Autodesk Inventor part; units mm, degrees
ref_plane "YZ Plane" through (0, 0, 0) normal (1, 0, 0) x (0, 1, 0)
ref_plane "XZ Plane" through (0, 0, 0) normal (0, 1, 0) x (-1, 0, 0)
ref_plane "XY Plane" through (0, 0, 0) normal (0, 0, 1) x (1, 0, 0)
sketch "Skizze1" plane through (0, 0, 0) normal (0, 1, 0) x (-1, 0, 0)
  line L0 (20.5, -10.1) -> (-20.5, -10.1)
  line L1 (-20.5, -10.1) -> (-20.5, 10.1)
  line L2 (-20.5, 10.1) -> (20.5, 10.1)
  line L3 (20.5, 10.1) -> (20.5, -10.1)
  line L4 (0, -23.94) -> (0, 23.94)
  line L5 (-40.6, 0) -> (40.6, 0)
  line L6 (29, -17.1) -> (-29, -17.1)
  line L7 (-29, -17.1) -> (-29, 17.1)
  line L8 (-29, 17.1) -> (29, 17.1)
  line L9 (29, 17.1) -> (29, -17.1)
  point P0 (0, 0)
  dimension "d0" = 41
  dimension "d3" = 20.2
  dimension "d7" = 58
  dimension "d8" = 7
extrude "Extrusion2" add sketch "Skizze1" along normal mid plane 4 contours L3 L5 L9 L6 L4 L0 | L4 L6 L7 L5 L1 L0 | L3 L2 L4 L8 L9 L5 | L5 L7 L8 L4 L2 L1
sketch "Skizze2" plane through (0, 2, 0) normal (0, 1, 0) x (1, 0, 0)
  circle A0 centre (-24, 5) radius 1.6
  circle A1 centre (-24, -5) radius 1.6
  line L0 (-29, 17.1) -> (-29, -17.1)
  line L1 (40.6, 0) -> (-40.6, 0)
  line L2 (0, 23.94) -> (0, -23.94)
  circle A2 centre (24, 5) radius 1.6
  circle A3 centre (24, -5) radius 1.6
  line L3 (-20.5, -10.1) -> (-20.5, 10.1)
  point P0 (0, 0)
  dimension "d11" = 3.2
  dimension "d12" = 3.2
  dimension "d15" = 10
  dimension "d16" = 5
  dimension "d58" = 3.5
  dimension "d59" = 3.5
extrude "Extrusion3" cut sketch "Skizze2" against normal up to surface (4 mm away)
sketch "Skizze3" plane through (0, 2, 0) normal (0, 1, 0) x (1, 0, 0)
  line L0 (-20.5, -10.1) -> (-20.5, 10.1)
  line L1 (-20.5, -0.75) -> (-27.5, -0.75)
  line L2 (-27.5, -0.75) -> (-27.5, 0.75)
  line L3 (-27.5, 0.75) -> (-20.5, 0.75)
  line L4 (-20.5, 0.75) -> (-20.5, -0.75)
  line L5 (40.6, 0) -> (-40.6, 0)
  line L6 (0, 23.94) -> (0, -23.94)
  line L7 (20.5, 10.1) -> (20.5, -10.1)
  line L8 (20.5, 0.75) -> (27.5, 0.75)
  line L9 (27.5, 0.75) -> (27.5, -0.75)
  line L10 (27.5, -0.75) -> (20.5, -0.75)
  line L11 (20.5, -0.75) -> (20.5, 0.75)
  point P0 (0, 0)
  dimension "d19" = 7
  dimension "d20" = 1.5
  dimension "d23" = 7
extrude "Extrusion4" cut sketch "Skizze3" against normal blind 2 contours L1 L2 L5 L0 | L5 L2 L3 L0
extrude "Extrusion5" cut sketch "Skizze3" against normal blind 2 contours L9 L10 L7 L5 | L5 L7 L8 L9
sketch "Skizze4" plane through (0, 0, 0) normal (0, 0, 1) x (1, 0, 0)
  line L0 (0, 34.5995) -> (0, -8.0999)
  line L1 (-12.8217, 0) -> (76.93, 0)
  line L2 (29, 2) -> (29, -2)
  line L3 (29, -2) -> (32, -2)
  line L4 (32, -2) -> (32, 19.216)
  line L5 (32, 19.216) -> (29, 19.216)
  line L6 (29, 19.216) -> (29, -2)
  line L7 (32, -2) -> (50.7939, 4.8404)
  line L8 (50.7939, 4.8404) -> (50.7939, 26.0564)
  line L9 (50.7939, 26.0564) -> (32, 19.216)
  line L10 (32, 15.858) -> (48.1939, 21.7521)
  line L11 (48.0492, 7.1994) -> (32, 1.358)
  line L12 (48.1939, 21.7521) -> (65.1083, 27.9084)
  line L13 (65.1083, 27.9084) -> (65.1083, 13.4084)
  line L14 (65.1083, 13.4084) -> (48.0492, 7.1994)
  line L15 (50.7939, 15.4484) -> (37.5768, 10.6378)
  line L16 (50.7939, 15.4484) -> (64.8591, 15.4484) construction
  point P0 (0, 0)
  point P1 (50.7939, 22.6984)
  point P2 (50.7939, 8.1984)
  dimension "d26" = 3
  dimension "d27" = 21.216
  dimension "d28" = 20
  dimension "d29" = 21.216
  dimension "d30" = 20
  dimension "d38" = 110
  dimension "d42" = 18
  dimension "d44" = 110
  dimension "d48" = 14.3145
  dimension "d66" = 14.5
  dimension "d67" = 160
extrude "Extrusion6" add sketch "Skizze4" along normal mid plane 34.2 contours L2 L6 L5 L4 L1 | L1 L4 L3 L2
sketch "Skizze6" plane through (0, 0, 0) normal (0, 0, 1) x (1, 0, 0)
  point P0 (0, 0)
extrude "Extrusion7" add sketch "Skizze4" along normal mid plane 20 contours L4 L11 L14 L8 L7 L1 | L1 L7 L4 | L4 L10 L12 L8 L14 L11 | L4 L9 L8 L12 L10
extrude "Extrusion9" add sketch "Skizze4" along normal mid plane 13.5 contours L8 L12 L13 L14
shell "Wandung2" thickness 2 removed faces 1 at (65.1083, 18.2418, -2.25)
fillet "Rundung1" radius 4 4 edges at (41.3969, 22.6362, 10) (41.3969, 22.6362, -10) (41.3969, 1.4202, -10) (41.3969, 1.4202, 10)
sketch "Skizze7" plane through (-29, -2, 17.1) normal (0, 0, 1) x (1, 0, 0)
  line L0 (-12.2, 2) -> (73.2, 2)
  line L1 (29, 25.4592) -> (29, -4.2432)
  line L2 (58, 4) -> (58, 21.216)
  line L3 (58, 21.216) -> (29, 4)
  line L4 (8.5, 4) -> (49.5, 4)
  line L5 (58, 4) -> (0, 4)
  line L6 (58, 4) -> (58, 21.216)
  point P0 (29, 2)
extrude "Extrusion10" add sketch "Skizze7" against normal blind 2
sketch "Skizze8" plane through (-29, -2, -17.1) normal (0, 0, -1) x (-1, 0, 0)
  line L0 (-29, -4.2432) -> (-29, 25.4592)
  line L1 (-73.2, 2) -> (12.2, 2)
  line L2 (-58, 4) -> (-58, 21.216)
  line L3 (-58, 21.216) -> (-29, 4)
  line L4 (-8.5, 4) -> (-49.5, 4)
  line L5 (-58, 4) -> (0, 4)
  line L6 (-58, 21.216) -> (-61, 21.216)
  line L7 (-58, 4) -> (-58, 21.216)
  point P0 (-29, 2)
extrude "Extrusion11" add sketch "Skizze8" against normal blind 2
sketch "Skizze9" plane through (0, 0, 6.75) normal (0, 0, 1) x (1, 0, 0)
  circle A0 centre (58.7939, 18.3602) radius 1.6
  line L0 (65.1083, 13.4084) -> (65.1083, 27.9084)
  line L1 (65.1083, 15.5368) -> (65.1083, 25.7801)
  line L2 (65.1083, 20.6584) -> (53.7155, 16.5118)
  line L3 (65.1083, 20.6584) -> (77.2323, 20.6584) construction
  line L4 (50.7939, 8.1984) -> (50.7939, 22.6984)
  point P0 (0, 0)
  dimension "d60" = 3.2
  dimension "d62" = 160
  dimension "d63" = 8
extrude "Extrusion12" cut sketch "Skizze9" against normal up to surface (13.5 mm away)
sketch "Skizze10" plane through (0, 0, 0) normal (0, 0, 1) x (1, 0, 0)
  line L0 (-46.9108, 47.129) -> (37.4559, 47.129)
  line L1 (37.4559, 47.129) -> (37.4559, -27.201)
  line L2 (37.4559, -27.201) -> (-46.9108, -27.201)
  line L3 (-46.9108, -27.201) -> (-46.9108, 47.129)
  point P0 (0, 0)
extrude "Extrusion13" cut sketch "Skizze10" along normal mid plane 50
properties part number "_3D-Druck"
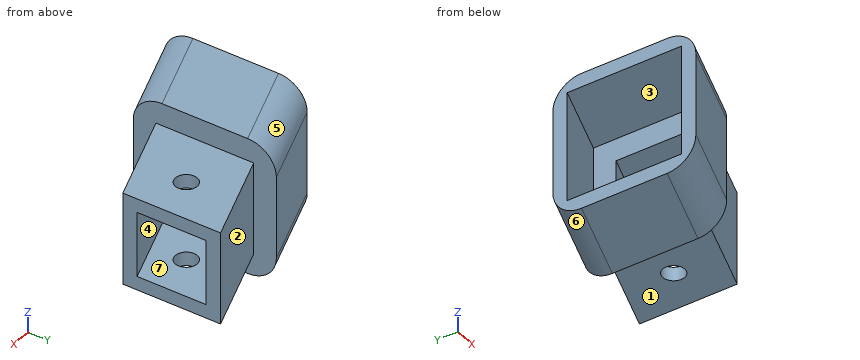
Can you work these out from the model? Positions are in its coordinate system, mm. Face numbers are marked on the shaded views. A direction names the side the tool comes from. Give positions to 0.01 mm unless a question says otherwise; leave off trailing zeros. Loops run counter-clockwise (first coordinate to the right, second up) from the corner with the lowest first, then second, coordinate; pieces in that order, holes last. Notation, with made-up numbers: (65, 60) -> (71, 60) arc R35 ccw to (71, 92) -> close; hole circle Ø2 at (73, 31). An arc over 180 degrees is marked (long way). Use one line per item in the form item = value.
1) If we section it at C-C (z = -5.25): Please give me the cut outline in (x, y), plus the area to 3 significant figures.
Answers:
outline = (37.46, -0.01) -> (50.79, 4.84) -> (50.79, 8.2) -> (65.11, 13.41) -> (65.11, 27.91) -> (50.79, 22.7) -> (50.79, 26.06) -> (37.46, 21.2) -> (37.46, 19.07) -> (48.79, 23.2) -> (48.79, 6.24) -> (37.46, 2.11) -> close; hole circle Ø3.2 at (58.79, 18.36)
area = 290 mm²
2) For the marked faces 1, 2, 3 and 4, which set-ups out of +Z, -Z, +X, -X, +Y, -Y let a thin tool reach every point of the face, with its end or its side?
Answers:
face_1 = -Z, +X, +Y, -Y
face_2 = +Z, -Z, +Y
face_3 = none
face_4 = -X
3) I need wall thicknesses on line 1 along Z through (x, y) = (52, 11.5); line 2 along Z through (x, y) = (39.25, 6.5); line 3 along Z through (x, y) = (63, 14). Which ranges of each line are inside material? Lowest first, please.
Answers:
line_1 = -6.75 to -4.75, 4.75 to 6.75
line_2 = -10 to -8, 8 to 10
line_3 = -6.75 to 6.75
4) If we section it at A-A (z = -2): Please give me the cut outline in (x, y), plus the area to 3 significant figures.
Answers:
outline = (37.46, -0.01) -> (50.79, 4.84) -> (50.79, 8.2) -> (65.11, 13.41) -> (65.11, 15.54) -> (48.79, 9.6) -> (48.79, 6.24) -> (37.46, 2.11) -> close; (37.46, 19.07) -> (48.79, 23.2) -> (48.79, 19.84) -> (65.11, 25.78) -> (65.11, 27.91) -> (50.79, 22.7) -> (50.79, 26.06) -> (37.46, 21.2) -> close
area = 131 mm²
5) Will these pins go through, and if not, where does the flat tip stop? pin 1 (1.5 mm diameter, centred on x = 43.5, z = 7, fed in from +Y); pin 2 (1.5 mm diameter, centred on x = 47.5, z = -6.5, fed in from -Y); pin 3 (7 mm diameter, centred on x = 54.5, y = 16.5, fed in from +Z).
Answers:
pin_1 = 23.59
pin_2 = 3.39
pin_3 = 6.75
6) We'd pull the mould along Z, two halves only. Please class the marked faces 5, 6 and 7: released by +Z, released by -Z, zero draft, split by the parting line, or undercut.
Answers:
face_5 = released by +Z
face_6 = released by -Z
face_7 = undercut
7) If we section it at B-B (x = 54.75): Please give me the cut outline in (y, z).
Answers:
outline = (9.64, -6.75) -> (24.14, -6.75) -> (24.14, 6.75) -> (9.64, 6.75) -> close; hole (11.77, -4.75) -> (22.01, -4.75) -> (22.01, 4.75) -> (11.77, 4.75) -> close
8) If we section it at D-D (x = 58.25): Please give me the cut outline in (y, z), plus the area to 3 significant figures.
Answers:
outline = (10.91, -6.75) -> (16.86, -6.75) -> (16.86, -4.75) -> (13.04, -4.75) -> (13.04, 4.75) -> (16.86, 4.75) -> (16.86, 6.75) -> (10.91, 6.75) -> close; (19.86, -6.75) -> (25.41, -6.75) -> (25.41, 6.75) -> (19.86, 6.75) -> (19.86, 4.75) -> (23.28, 4.75) -> (23.28, -4.75) -> (19.86, -4.75) -> close
area = 86.4 mm²
